Here's how the part is built. I have some questions about the finished solid (model axes, mm). A direction names the side the tool comes from. Coordinates: 2 decimals unless noted, no trailing zeros. Order: outer loops, then holes, each group sorted by start corner. A loop starts at its lowest first (then second) coordinate and runs counter-clockwise, first axis right, second up. Notation, with made-up numbers: (-29, -33.75) - (-1, -33.75) arc R10 cw to (-1, -28.75) - close; hole circle Ø1 at (-3, 26.5). An arc over 180 degrees is marked (long way). Answer in a Markdown table with one row per item. Add a question column.
Item 1: If I drill on line 1 along Y through (x, z) = (0, -25.25); line 2 along Z through (x, y) = (0, 0.35), over which ranges is the centre line in solid material (lowest first)? Write a range as from..to.
Item 2: I want a section at B-B (z = -11.5). Please give me the cut outline in (x, y).
Item 3: Thinking about a two-plate mould opening in X: for faces 3 (the cylindrical face through (-0.217, 0.254, 0.976)), 4 (the cylindrical face through (-0.27, 6.22, -18.44)), which applies, +X half, -X half, draft (parallel to the pull), parting line (faces both ways), or undercut?
Item 4: I want a section at A-A (x = 0). Please give me the cut outline in (y, z), plus the area to 3 significant figures.
Item 5: On a 3-axis mill with a long thin cutter (end or side, diameter ignored), from which of +Z, -Z, +X, -X, +Y, -Y can I reach the whole of each face in a straight line? I mean faces 1 (the cylindrical face through (-0.27, 0.25, 1.22)), 2 (the cylindrical face through (0, 4, -18)). Say none if no direction works.
Item 6: Will these pins go through, and if not, where does the flat tip stop? pin 1 Ø1.5 at (x, y) = (-1, 1) entering from -Z; pin 2 Ø1 at (x, y) = (-0.5, 1) entering from -Z.
```python
from build123d import *

# Parameters (mm, degrees)
SKIZZE2_R   = 1.25
SKIZZE2_R_2 = 1


with BuildPart() as part:
    # Austragung1: sweep along a path in Skizze1
    with BuildLine(Plane(origin=(0, 0, 0), x_dir=(0, 0, -1), z_dir=(1, 0, 0))) as austragung1_path:
        Line((0, 0), (0, 0.5))
        ThreePointArc((0, 0.5), (1.318019485, 3.681980515), (4.5, 5))
        Line((4.5, 5), (32, 5))
    # Skizze2 → Austragung1 (sweep)
    with BuildSketch(Plane(origin=(0, 0, 0), x_dir=(1, 0, 0), z_dir=(0, 1, 0))):
        Circle(SKIZZE2_R)
        Circle(SKIZZE2_R_2, mode=Mode.SUBTRACT)
    sweep(path=austragung1_path.line)


solid = part.part
```
Values follow:
| question | item | result |
|---|---|---|
| 1 | line 1 | y = 3.75..4, 6..6.25 |
| 1 | line 2 | z = -1.25..-1, 1..1.25 |
| 2 | outline | circle Ø2.5 at (0, 5); hole circle Ø2 at (0, 5) |
| 3 | face 3 | undercut |
| 3 | face 4 | parting line |
| 4 | outline | (0, -1.25) - (0.5, -1.25) arc R3.25 cw to (3.75, -4.5) - (3.75, -32) - (4, -32) - (4, -4.5) arc R3.5 ccw to (0.5, -1) - (0, -1) - close; (0, 1) - (0.5, 1) arc R5.5 cw to (6, -4.5) - (6, -32) - (6.25, -32) - (6.25, -4.5) arc R5.75 ccw to (0.5, 1.25) - (0, 1.25) - close |
| 4 | area | 17.5 mm^2 |
| 5 | face 1 | -Y |
| 5 | face 2 | -Z |
| 6 | pin 1 | stops at z = -1.32 |
| 6 | pin 2 | stops at z = -1.36 |
